Geometry check sheet. Reference: drawing and pictorial views, mm from the part's lowest x, y, z. A direction names the side the tool comes from. Give positions to 0.01 mm unless a question says otherwise; leave off trailing zeros. Write each loop counter-clockwise with the first axis right and the second up, starting at its lowest first coordinate (ties: lowest second). Pieces come first, ordered by that corner, then holes. Notation, with made-up numbers: M 9,33 L 60,33 A34 cw 60,71 Z; hole C -28,26 d1. An arc over 180 degrees is marked long. One line per item, written item: value. Start each with the question number.
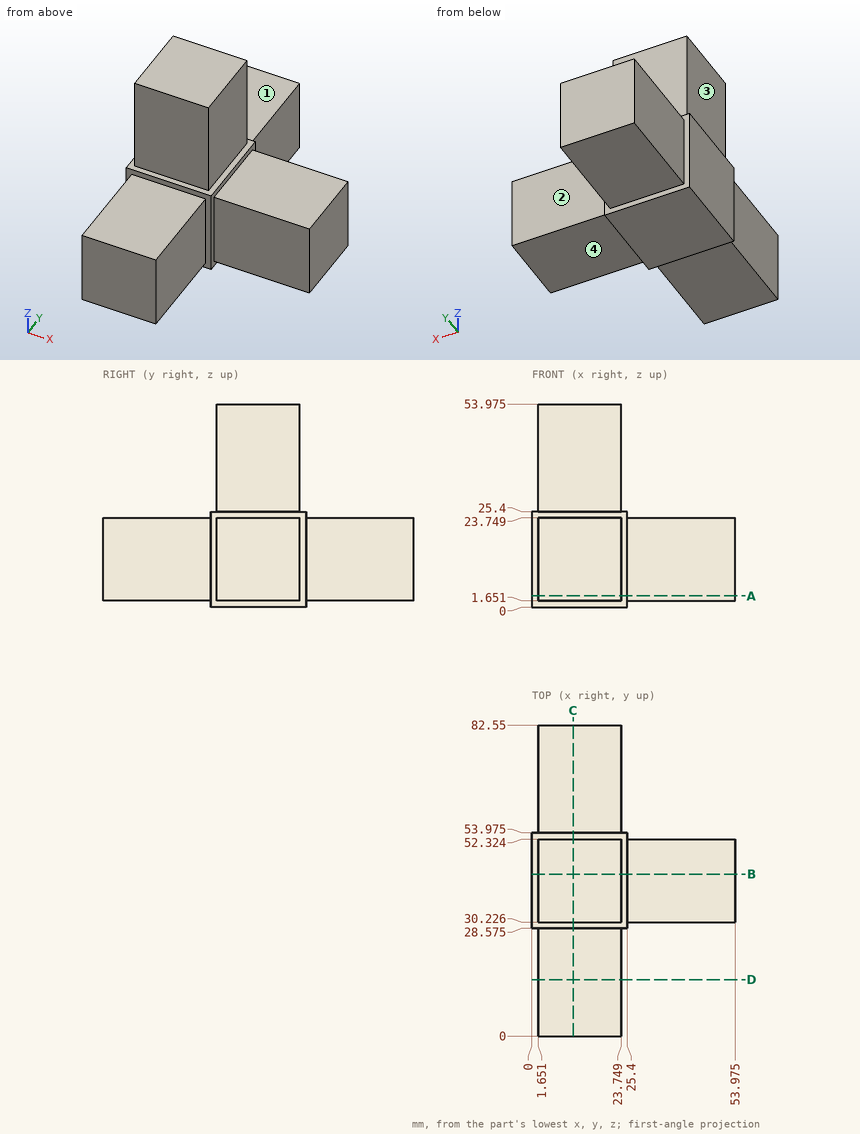
1) Cross-section at D-D (y = 15). Record the boundary of the cut face in (x, z).
2) Cross-section at A-A (z = 3). Record the boundary of the cut face in (x, y) (3 decimals), plus the area to 3 significant figures.
3) Cross-section at C-C (x = 11). Record the boundary of the cut face in (y, z) (3 decimals).
4) Material ranges on L1, parallel to X at y = 36, z = 41.5; L2, parallel to Y at x = 3, z = 45, recorded low to high. Write a range as from..to.
5) Gauge pin test, flat ends, axial feed: pin 1 (17.5 mm diameter, centred on y = 75, z = 9.5, fed in from -X); pin 2 (11 mm diameter, centred on x = 15, y = 13, fed in from -Z); pin 3 (2 mm diameter, centred on x = 9.5, z = 29, fed in from +Y); pin 4 (8 mm diameter, centred on x = 30, y = 19.5, fed in from +Z). Record the tip position at first contact, or that the pin passes through.
6) Cross-section at B-B (y = 43). Record the boundary of the cut face in (x, z) (3 decimals), plus the area to 3 significant figures.
7) Tool access check on the marked faces 1, 2, 3 and 4. Record the directions out of +Z, -Z, +X, -X, +Y, -Y that give a thin tool (end or side, any length) a straight path to the whole face; none if there is none.
Data:
1. outline: M 1.65,1.65 L 23.75,1.65 L 23.75,23.75 L 1.65,23.75 Z
2. outline: M 0,28.575 L 1.651,28.575 L 1.651,0 L 23.749,0 L 23.749,28.575 L 25.4,28.575 L 25.4,30.226 L 53.975,30.226 L 53.975,52.324 L 25.4,52.324 L 25.4,53.975 L 23.749,53.975 L 23.749,82.55 L 1.651,82.55 L 1.651,53.975 L 0,53.975 Z
2. area: 2,540 mm2
3. outline: M 0,1.651 L 28.575,1.651 L 28.575,0 L 53.975,0 L 53.975,1.651 L 82.55,1.651 L 82.55,23.749 L 53.975,23.749 L 53.975,25.4 L 52.324,25.4 L 52.324,53.975 L 30.226,53.975 L 30.226,25.4 L 28.575,25.4 L 28.575,23.749 L 0,23.749 Z
4. L1: x = 1.65..23.75
4. L2: y = 30.23..52.32
5. pin 1: stops at x = 1.65
5. pin 2: stops at z = 1.65
5. pin 3: stops at y = 52.32
5. pin 4: passes through
6. outline: M 0,0 L 25.4,0 L 25.4,1.651 L 53.975,1.651 L 53.975,23.749 L 25.4,23.749 L 25.4,25.4 L 23.749,25.4 L 23.749,53.975 L 1.651,53.975 L 1.651,25.4 L 0,25.4 Z
6. area: 1,910 mm2
7. face 1: +Z, +X, -X, +Y
7. face 2: +Z, -Z, +X, +Y
7. face 3: +Z, -X, +Y, -Y
7. face 4: -Z, +X, +Y, -Y
